Can you work these out from the drawing? Everything is in mm from the part's minimum corner. Coordinates: 2 decimals unless noted, no trailing zeros. Loops run counter-clockwise (first coordinate to the right, second up) from the corner with the lowest first, then second, coordinate; pieces in that order, holes last. Notation, with made-up numbers: (6.25, -40) - (11.25, -40) arc R19 ccw to (11.25, -34) - close; hole circle Ø2 at (-16, -2.5). An arc over 180 degrees is marked (long way). Put each result on its own line as item: value. Start each with the question number.
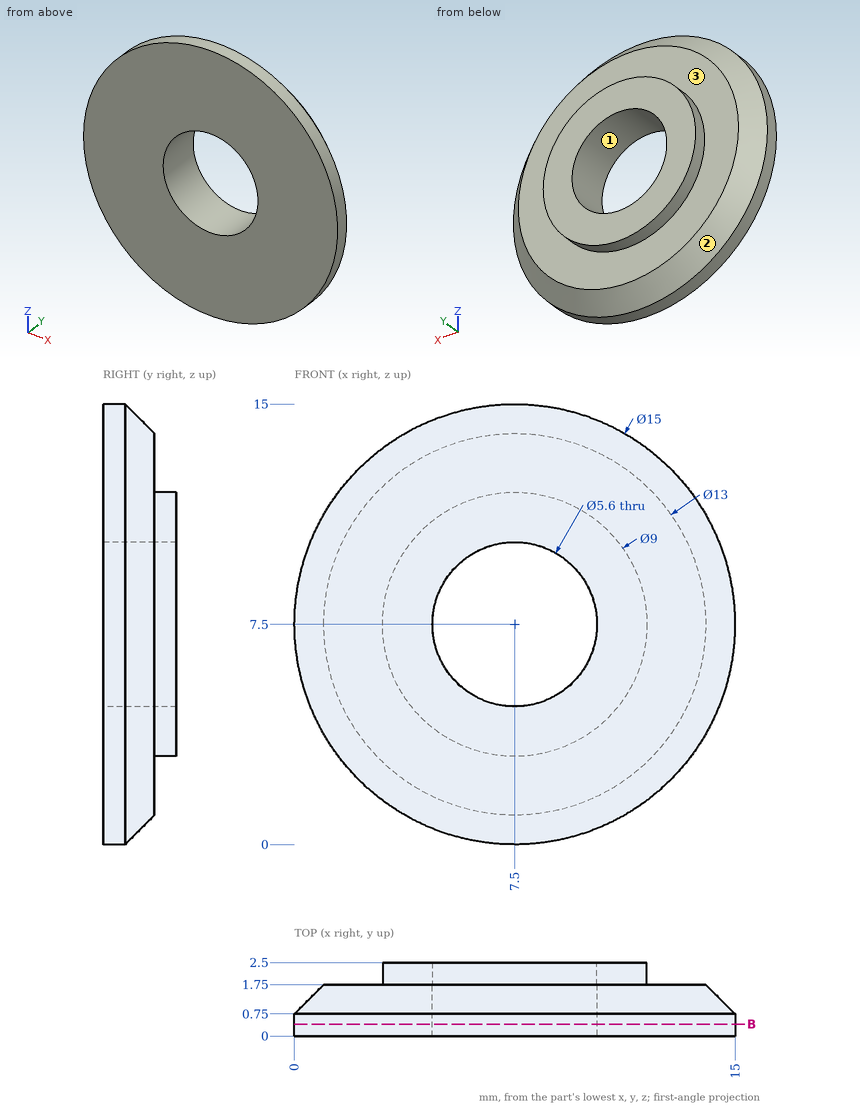
Q1. Will these pins go through, and if not, where does the flat tip stop? pin 1 (2 mm diameter, centred on x = 11.5, z = 3, fed in from +Y); pin 2 (1.5 mm diameter, centred on x = 9, y = 1, fed in from -Z); pin 3 (1 mm diameter, centred on x = 11, y = 1.5, fed in from +Z).
Q2. Please list where these lines run through material, in increasing order: line 1 along Z through (x, y) = (7.5, 1.9); line 2 along Z through (x, y) = (7.5, 0.5). Write a range as [from, to].
Q3. We'd pull the mould along X, two halves only. Please class the marked faces 1, 2 and 3: released by +X, released by -X, zero draft, split by the parting line, or undercut.
Q4. I want a section at B-B on y = 0.4. List the corners of the cut face in (x, z) for me, and give its area (3 significant figures).
Calculated:
1. pin 1: y = 1.75
1. pin 2: z = 0.04
1. pin 3: z = 13.91
2. line 1: [3, 4.7], [10.3, 12]
2. line 2: [0, 4.7], [10.3, 15]
3. face 1: undercut
3. face 2: split by the parting line
3. face 3: zero draft
4. outline: circle Ø15 at (7.5, 7.5); hole circle Ø5.6 at (7.5, 7.5)
4. area: 152 mm2
